from build123d import *

# Parameters (mm, degrees)
F3_DEPTH       = 18
F4_DEPTH       = 14
F5_D           = 8.4
F5_CBORE_D     = 14.25
F5_CBORE_DEPTH = 8


with BuildPart() as f3:
    # F2 (on Right) → F3 (new body)
    with BuildSketch(Plane.YZ):
        Polygon((-194.2, 232), (-225, 232), (-225, 87.6), (207, 87.6), (207, 78.6), (225, 78.6), (225, 159.8), (207, 159.8), (207, 191.7), (196.5, 191.7), (196.5, 188.9), (187.5, 188.9), (187.5, 191.7), (177, 191.7), (176, 191.7), (176, 200.1), (177, 200.1), (187.5, 200.1), (187.5, 202.9), (196.5, 202.9), (196.5, 200.1), (207, 200.1), (207, 232), (4.2, 232), (4.2, 221.5), (7, 221.5), (7, 212.5), (4.2, 212.5), (4.2, 201), (-4.2, 201), (-4.2, 212.5), (-7, 212.5), (-7, 221.5), (-4.2, 221.5), (-4.2, 232), (-185.8, 232), (-185.8, 221.5), (-183, 221.5), (-183, 212.5), (-185.8, 212.5), (-185.8, 202), (-185.8, 201), (-194.2, 201), (-194.2, 202), (-194.2, 212.5), (-197, 212.5), (-197, 221.5), (-194.2, 221.5), align=None)
    extrude(amount=-F3_DEPTH)



with BuildPart() as f3b:
    # F2 (on Right) → F3, piece 2 (new body)
    with BuildSketch(Plane.YZ):
        Polygon((207, 69.6), (-225, 69.6), (-225, -156), (207, -156), (207, -128.6), (196.5, -128.6), (196.5, -131.4), (187.5, -131.4), (187.5, -128.6), (176, -128.6), (176, -120.2), (187.5, -120.2), (187.5, -117.4), (196.5, -117.4), (196.5, -120.2), (207, -120.2), (207, -83.8), (225, -83.8), (225, -2.6), (207, -2.6), align=None)
    extrude(amount=-F3_DEPTH)


with BuildPart() as f3c:
    # F2 (on Right) → F3, piece 3 (new body)
    with BuildSketch(Plane.YZ):
        with BuildLine():
            Line((207, -174), (-225, -174))
            Line((-225, -174), (-225, -250))
            Line((-225, -250), (-155, -250))
            ThreePointArc((-155, -250), (-140.3553390593, -214.6446609407), (-105, -200))
            Line((-105, -200), (105, -200))
            ThreePointArc((105, -200), (140.3553390593, -214.6446609407), (155, -250))
            Line((155, -250), (225, -250))
            Line((225, -250), (225, -165))
            Line((225, -165), (207, -165))
            Line((207, -165), (207, -174))
        make_face()
    extrude(amount=-F3_DEPTH)


with BuildPart() as f3_1:
    add(f3.part)

    add(f3b.part)  # F4 merges F3b

    add(f3c.part)  # F4 merges F3c
    # F2 (on Right) → F4 (join)
    with BuildSketch(Plane.YZ):
        Polygon((207, 87.6), (-225, 87.6), (-225, 69.6), (207, 69.6), (207, 78.6), align=None)
        Polygon((207, -156), (-225, -156), (-225, -174), (207, -174), (207, -165), align=None)
    extrude(amount=-F4_DEPTH)

    # F5 (through all)
    with Locations(Plane.YZ):
        with Locations((-190, 78.6), (0, 78.6), (0, -165), (-190, -165)):
            CounterBoreHole(F5_D / 2, F5_CBORE_D / 2, F5_CBORE_DEPTH)


solid = f3_1.part
Build history of the part. All positions in model axes, mm. A direction names the side the tool comes from. Round coordinates to 2 decimals unless told otherwise and drop trailing zeros. Write each loop counter-clockwise with the first axis right and the second up, starting at its lowest first coordinate (ties: lowest second). Pieces come first, ordered by that corner, then holes. Notation, with made-up numbers: (54.25, -13) -> (64.25, -13) arc R15 cw to (64.25, 5) -> close; hole circle Ø5 at (15, -19.5). An arc over 180 degrees is marked (long way). Write item = value, one per line.
(1) Band-saw the part on B-B (x = -4.5). State how many separate pieces and enclosed holes the cut face has, then the cut area to 3 significant figures.
Answer:
separate_pieces = 1
enclosed_holes = 4
area = 196,000 mm2
(2) Flat gauge pins, fed straight in: pin 1 (3 mm diameter, centred on x = -4, z = 41, fed in from +Y); pin 2 (3 mm diameter, centred on x = -5, y = -6, fed in from -Z); pin 3 (11.5 mm diameter, centred on y = -190, z = -165, fed in from -X). Where does each tip first touch, or does it go through?
Answer:
pin_1 = 207
pin_2 = -200
pin_3 = -14
(3) Probe L1, parallel to Z at x = -3.75, y = -190 (3 decimals); L2, parallel to Z at x = -9.8, y = -190; L3, parallel to Z at x = -15.25, y = 195. List the from-to ranges inside material, lowest first.
Answer:
L1 = -250 to -172.125, -157.875 to 71.475, 85.725 to 201
L2 = -250 to -169.2, -160.8 to 74.4, 82.8 to 201
L3 = -250 to -174, -156 to -131.4, -117.4 to 69.6, 87.6 to 188.9, 202.9 to 232
(4) Band-saw the part on A-A (y = -169). Give the cut face in (x, z).
Answer:
outline = (-18, -250) -> (0, -250) -> (0, 232) -> (-18, 232) -> (-18, 87.6) -> (-14, 87.6) -> (-14, 69.6) -> (-18, 69.6) -> (-18, -156) -> (-14, -156) -> (-14, -174) -> (-18, -174) -> close
(5) Tool access for faces 1 (the face through (-3.944, -0.928, 85.664)), 2 (the face through (-9, 202, -128.6)), 3 (the face through (-9, 216, 159.8)), 4 (the face through (-9, -194.2, 227)): list every direction of +Z, -Z, +X, -X, +Y, -Y with a clear straight run to the whole face (end or side of a thin tool).
Answer:
face_1 = +X
face_2 = +X, -X, +Y
face_3 = +Z, +X, -X, +Y
face_4 = +Z, +X, -X
(6) Band-saw the part on C-C (z = 52). Give the cut face in (x, y).
Answer:
outline = (-18, -225) -> (0, -225) -> (0, 207) -> (-18, 207) -> close
(7) Two-plate mould, pull along Z, no slides. Class faces 5 (the face through (-9, 190, -250)), 6 (the face through (-9, -94, 232)), 7 (the face through (-18, -3, -42)), 8 (the face through (-9, 182, -120.2)): pulls with the +Z half, pulls with the -Z half, needs draft (parallel to the pull), parting line crosses it, or undercut.
Answer:
face_5 = pulls with the -Z half
face_6 = pulls with the +Z half
face_7 = needs draft
face_8 = undercut
